from build123d import *

# Parameters (mm, degrees)
ESBO_O1_W                = 15.15
ESBO_O1_H                = 30.65
ESBO_O1_R                = 1.55
RESSALTO_EXTRUS_O1_DEPTH = 1.55
ESBO_O2_W                = 6.85
ESBO_O2_H                = 6.85
RESSALTO_EXTRUS_O2_DEPTH = 6.45
ESBO_O3_R                = 1.65
CORTE_EXTRUS_O1_DEPTH    = 0.5
ESBO_O4_W                = 7.3
ESBO_O4_H                = 2.5
RESSALTO_EXTRUS_O3_DEPTH = 4.05
RESSALTO_EXTRUS_O5_DEPTH = 7.398508
ESBO_O12_W               = 1.34798559
ESBO_O12_H               = 5.991047065
ESBO_O12_W_2             = 0.998507844
ESBO_O12_W_3             = 2
CORTE_EXTRUS_O2_DEPTH    = 10
ESBO_O9_R                = 1.55
CORTE_EXTRUS_O3_DEPTH    = 0.1
ESBO_O15_R               = 0.297205441
ESBO_O15_R_2             = 0.285630525
RESSALTO_EXTRUS_O6_DEPTH = 2


with BuildPart() as part:
    # Esboço1 → Ressalto-extrusão1 (new body)
    with BuildSketch(Plane.XY):
        Rectangle(ESBO_O1_W, ESBO_O1_H)
        with Locations(Location((0, -6.025, 0), (0, 0, 180))):
            Circle(ESBO_O1_R, mode=Mode.SUBTRACT)
    extrude(amount=RESSALTO_EXTRUS_O1_DEPTH)

    # Esboço2 → Ressalto-extrusão2 (add)
    with BuildSketch(Plane.XY):
        with Locations((3.95, 1.7)):
            Rectangle(ESBO_O2_W, ESBO_O2_H)
    extrude(amount=RESSALTO_EXTRUS_O2_DEPTH)

    # Esboço3 → Corte-extrusão1 (cut)
    with BuildSketch(Plane.XY.offset(6.45)):
        with Locations((3.95, 1.7)):
            Circle(ESBO_O3_R)
        with BuildLine():
            Line((3.7, 1.95), (2.420294146, 1.95))
            ThreePointArc((2.420294146, 1.95), (2.853984489, 2.796015511), (3.7, 3.229705854))
            Line((3.7, 3.229705854), (3.7, 1.95))
        make_face(mode=Mode.SUBTRACT)
        with BuildLine():
            Line((5.479705854, 1.45), (4.2, 1.45))
            Line((4.2, 1.45), (4.2, 0.170294146))
            ThreePointArc((4.2, 0.170294146), (5.046015511, 0.603984489), (5.479705854, 1.45))
        make_face(mode=Mode.SUBTRACT)
        with BuildLine():
            Line((5.479705854, 1.95), (4.2, 1.95))
            Line((4.2, 1.95), (4.2, 3.229705854))
            ThreePointArc((4.2, 3.229705854), (5.046015511, 2.796015511), (5.479705854, 1.95))
        make_face(mode=Mode.SUBTRACT)
        with BuildLine():
            Line((3.7, 1.45), (3.7, 0.170294146))
            ThreePointArc((3.7, 0.170294146), (2.853984489, 0.603984489), (2.420294146, 1.45))
            Line((2.420294146, 1.45), (3.7, 1.45))
        make_face(mode=Mode.SUBTRACT)
    extrude(amount=-CORTE_EXTRUS_O1_DEPTH, mode=Mode.SUBTRACT)

    # Esboço4 → Ressalto-extrusão3 (add)
    with BuildSketch(Plane.XY):
        with Locations((0, -13.975)):
            Rectangle(ESBO_O4_W, ESBO_O4_H)
    extrude(amount=RESSALTO_EXTRUS_O3_DEPTH)

    # Esboço11 → Ressalto-extrusão5 (add)
    with BuildSketch(Plane.ZY.offset(3.65)):
        with BuildLine():
            Line((4.05, -14.175), (4.467357012, -14.175))
            ThreePointArc((4.467357012, -14.175), (4.679489046, -14.262867966), (4.767357012, -14.475))
            Line((4.767357012, -14.475), (4.767357012, -18.595051461))
            Line((4.767357012, -18.595051461), (5.167357012, -18.595051461))
            Line((5.167357012, -18.595051461), (5.167357012, -14.475))
            ThreePointArc((5.167357012, -14.475), (4.962331759, -13.980025253), (4.467357012, -13.775))
            Line((4.467357012, -13.775), (4.05, -13.775))
            Line((4.05, -13.775), (4.05, -14.175))
        make_face()
    extrude(amount=-RESSALTO_EXTRUS_O5_DEPTH)

    # Esboço12 → Corte-extrusão2 (cut)
    with BuildSketch(Plane.XY.offset(4.05)):
        with Locations((-3.423992795, -16.372351479)):
            Rectangle(ESBO_O12_W, ESBO_O12_H)
        with Locations((3.249253922, -16.372351479)):
            Rectangle(ESBO_O12_W_2, ESBO_O12_H)
        with Locations((-1.25, -16.372351479)):
            Rectangle(ESBO_O12_W_3, ESBO_O12_H)
        with Locations((1.25, -16.372351479)):
            Rectangle(ESBO_O12_W_3, ESBO_O12_H)
    extrude(amount=CORTE_EXTRUS_O2_DEPTH, mode=Mode.SUBTRACT)

    # Esboço9 → Corte-extrusão3 (cut)
    with BuildSketch(Plane.XY.offset(6.45)):
        with Locations((3.95, 1.7)):
            Circle(ESBO_O9_R)
    extrude(amount=-CORTE_EXTRUS_O3_DEPTH, mode=Mode.SUBTRACT)

    # Esboço15 → Ressalto-extrusão6 (add)
    with BuildSketch(Plane.XY.offset(1.55)):
        with Locations(Location((1.7, 13.325, 0), (0, 0, 180))):
            Circle(ESBO_O15_R)
        with Locations(Location((-1.7, 13.325, 0), (0, 0, 180))):
            Circle(ESBO_O15_R_2)
    extrude(amount=RESSALTO_EXTRUS_O6_DEPTH)


solid = part.part
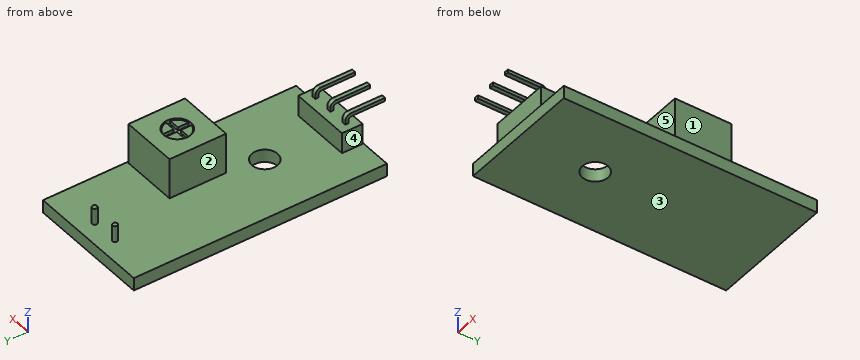
Source: CAD feature listing. Evaluate the final solid. Frame: model axes, mm. Face numbers are marked on the shaded views. A direction names the side the tool comes from. Coordinates: 2 decimals unless noted, no trailing zeros. Loops run counter-clockwise (first coordinate to the right, second up) from the corner with the lowest first, then second, coordinate; pieces in that order, holes last. Notation, with made-up numbers: M -39.75,64 L -18.75,64 A26 cw -18.75,86 Z; hole C -10,-3 d4. An arc over 180 degrees is marked long. Answer in a Markdown table with one row per item.
Q1. Section A-A on x = 6.5. Return the cut outline in (y, z) (3 decimals), plus the area to 3 significant figures.
Answers below:
| item | result |
|---|---|
| outline | M -15.325,0 L 15.325,0 L 15.325,1.55 L 5.125,1.55 L 5.125,6.45 L -1.725,6.45 L -1.725,1.55 L -15.325,1.55 Z |
| area | 81.1 mm^2 |
Q2. Section D-D on y = -11.5. Return the cut outline in (x, z) (3 decimals), plus the area to 3 significant figures.
Answers below:
| item | result |
|---|---|
| outline | M -7.575,0 L 7.575,0 L 7.575,1.55 L -7.575,1.55 Z |
| area | 23.5 mm^2 |
Q3. Section C-C on z = 1. Return the cut outline in (x, y) (3 decimals).
Answers below:
| item | result |
|---|---|
| outline | M -7.575,-15.325 L 7.575,-15.325 L 7.575,15.325 L -7.575,15.325 Z; hole C 0,-6.025 d3.1 |
Q4. Set-up query: the marked faces 1, 2 and 3. Return all of +Z, -Z, +X, -X, +Y, -Y with unobstructed straight access to the full face (end or side cutting, diameter ignored); none if empty.
Answers below:
| item | result |
|---|---|
| face 1 | +Z, +X, +Y, -Y |
| face 2 | +Z, -X, +Y |
| face 3 | -Z, +X, -X, +Y, -Y |
Q5. Ray query, probe 1 along Y at (x, z) = (3.95, 6.3) (3 decimals); probe 2 along Y at (x, z) = (0, 0.65) (3 decimals); probe 3 along Y at (x, z) = (-1.75, 4) (3 decimals). Return the intervals inside material, ascending. Write a range as from..to.
Answers below:
| item | result |
|---|---|
| probe 1 | y = -1.725..0.05, 3.35..5.125 |
| probe 2 | y = -15.325..-7.575, -4.475..15.325 |
| probe 3 | y = -15.225..-12.725 |
Q6. Section B-B on x = 1. Return the cut outline in (y, z) (3 decimals), plus the area to 3 significant figures.
Answers below:
| item | result |
|---|---|
| outline | M -15.325,0 L -7.209,0 L -7.209,1.55 L -12.725,1.55 L -12.725,4.05 L -15.225,4.05 L -15.225,1.55 L -15.325,1.55 Z; M -4.841,0 L 15.325,0 L 15.325,1.55 L 5.125,1.55 L 5.125,6.45 L -1.725,6.45 L -1.725,1.55 L -4.841,1.55 Z |
| area | 83.7 mm^2 |
Q7. First-contact query: pin 1 (1 mm diameter, centred on y = 12, z = 5.5, fed in from +X); pin 2 (2.5 mm diameter, centred on y = 0.5, z = 3.5, fed in from -X) (3 decimals); pin 3 (1.5 mm diameter, centred on x = 3.5, z = 3.5, fed in from +Y) (3 decimals); pin 4 (1.2 mm diameter, centred on x = 1.5, z = 3, fed in from -Y) (3 decimals). Flat tips, straight axial feed; report the tip coordinate or a pass-through.
Answers below:
| item | result |
|---|---|
| pin 1 | passes through |
| pin 2 | stops at x = 0.525 |
| pin 3 | stops at y = 5.125 |
| pin 4 | stops at y = -15.225 |
Q8. Draft query along Y for the marked faces 4 and 5. Return one class per face: pulls with the +Y half, pulls with the -Y half, needs draft (parallel to the pull), parting line crosses it, or undercut.
Answers below:
| item | result |
|---|---|
| face 4 | needs draft |
| face 5 | undercut |
